Geometry: see drawing. Coordinates: mm, zero at the bounding-box minimum. Give positions to 0.01 mm unless a question says otherwise; leave off trailing zeros. Write each loop counter-clockwise with the first axis right and the second up, starting at its lowest first coordinate (ties: lowest second). Pieces come first, ordered by that corner, then holes. Notation, with made-up numbers: (75, 9) -> (112, 9) arc R13 ccw to (112, 14) -> close; hole circle Ø6 at (51, 36). An arc over 180 degrees is marked (long way). Write item = value, one per line.
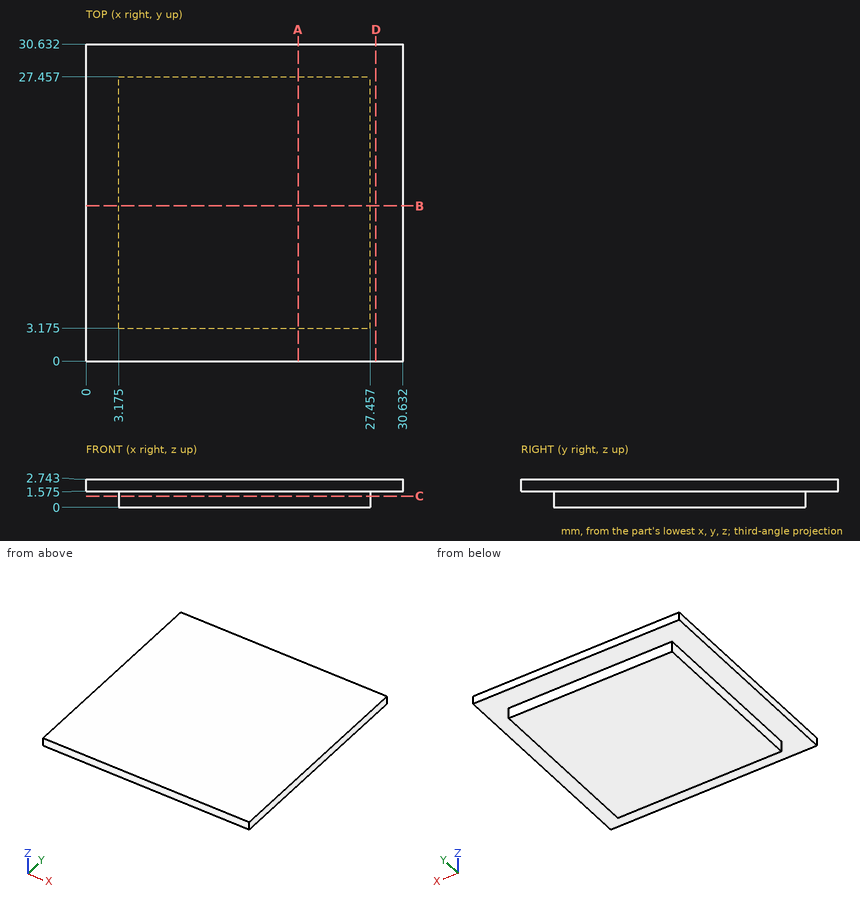
(1) Section query C-C (z = 1.1). Return loops of the section in (x, y) (1 decimal).
Values follow:
outline = (3.2, 3.2) -> (27.5, 3.2) -> (27.5, 27.5) -> (3.2, 27.5) -> close
(2) Section query A-A (x = 20.5). Return loops of the section in (y, z) (1 decimal).
Values follow:
outline = (0, 1.6) -> (3.2, 1.6) -> (3.2, 0) -> (27.5, 0) -> (27.5, 1.6) -> (30.6, 1.6) -> (30.6, 2.7) -> (0, 2.7) -> close
(3) Section query D-D (x = 28). Return loops of the section in (y, z) (1 decimal).
Values follow:
outline = (0, 1.6) -> (30.6, 1.6) -> (30.6, 2.7) -> (0, 2.7) -> close
(4) First-contact query: pin 1 (1.5 mm diameter, centred on x = 15.5, y = 4, fed in from -Z); pin 2 (0.5 mm diameter, centred on y = 10.5, z = 1, fed in from +X); pin 3 (0.8 mm diameter, centred on y = 14, z = 1, fed in from -X) (3 decimals). Flat tips, straight axial feed; report the tip coordinate or a pass-through.
Values follow:
pin_1 = 0
pin_2 = 27.46
pin_3 = 3.175
(5) Material intervals for line 1 (Y direction, x = 3.5, z = 1.25) (1 decimal); line 2 (Z direction, x = 6.5, y = 3) (1 decimal), sorted ascending.
Values follow:
line_1 = 3.2 to 27.5
line_2 = 1.6 to 2.7
